For this review, use the dimensioned drawing (mm, ordinates from the lowest corner) and the shaded views. A direction names the side the tool comes from. Coordinates: 2 decimals unless noted, no trailing zeros. Order: outer loops, then holes, each group sorted by start corner. A loop starts at its lowest first (then second) coordinate and runs counter-clockwise, first axis right, second up. Notation, with made-up numbers: M 6,80 L 23,80 A20 cw 23,112 Z; hole C -39.75,47 d11. An arc over 180 degrees is marked long. Answer in a Markdown table with one row per item.
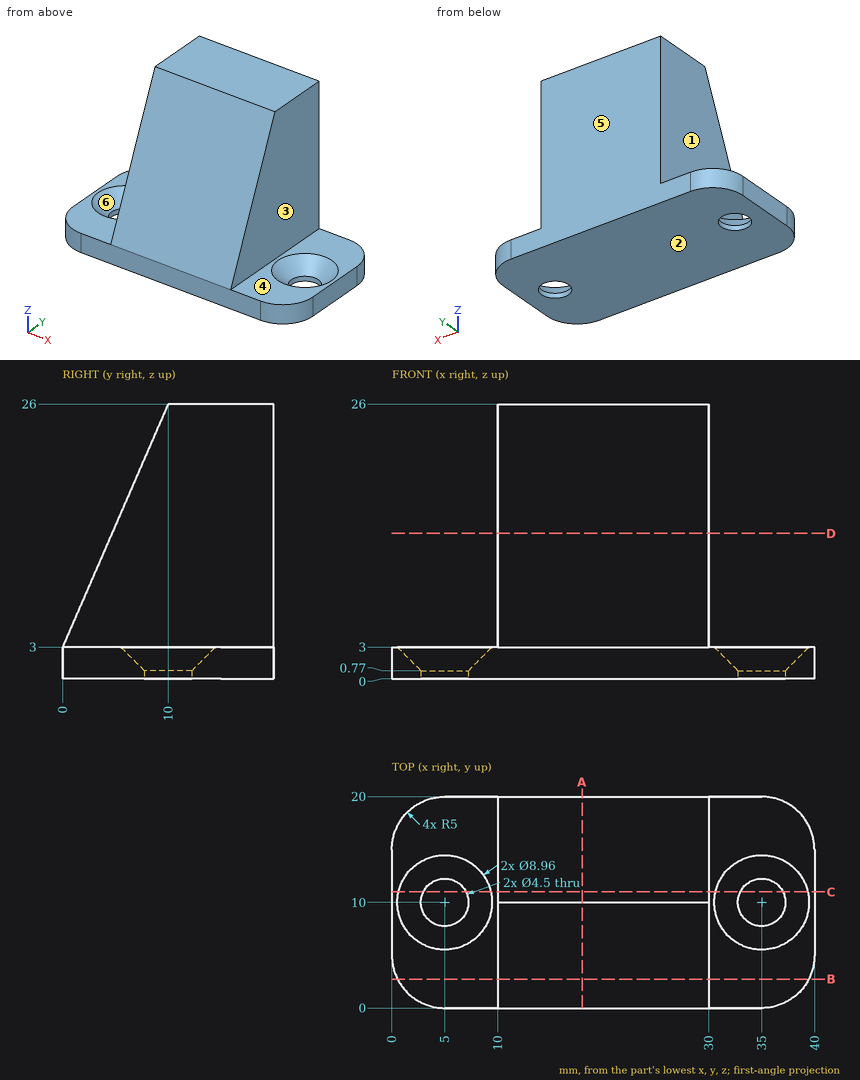
(1) Draft analysis for pull direction Y (two halves, no side actions). For the marked faces 4, 5 and 6, state which applies: pulls with the +Y half, pulls with the -Y half, needs draft (parallel to the pull), parting line crosses it, or undercut.
Return value:
| item | result |
|---|---|
| face 4 | needs draft |
| face 5 | pulls with the +Y half |
| face 6 | undercut |
(2) Add section A-A, the plane x = 18. Give the boundary of the cut face in (y, z), and give its area (3 significant figures).
Return value:
| item | result |
|---|---|
| outline | M 0,0 L 20,0 L 20,26 L 10,26 L 0,3 Z |
| area | 405 mm2 |
(3) For the marked faces 1, 2 and 3, list the 3-axis set-ups (+Z, -Z, +X, -X, +Y, -Y) from which the entire face can be reached by the end or side of a thin tool; tool diameter is ignored.
Return value:
| item | result |
|---|---|
| face 1 | +Z, -X, +Y, -Y |
| face 2 | -Z, +X, -X, +Y, -Y |
| face 3 | +Z, +X, +Y, -Y |
(4) Add section D-D, the plane z = 13.75. Give the boundary of the cut face in (x, y), and give its area (3 significant figures).
Return value:
| item | result |
|---|---|
| outline | M 10,4.67 L 30,4.67 L 30,20 L 10,20 Z |
| area | 307 mm2 |
(5) Insertion check: pin 1 Ø12 at (x, z) = (8, 11.5) entering from +Y; pin 2 Ø7 at (x, y) = (5, 10) entering from +Z; pin 3 Ø10 at (y, z) = (9.5, 18.5) entering from -X; pin 4 Ø6 at (x, y) = (35, 10) entering from +Z. Each pin has a flat end and moves straight along its axis. Give the tip position at first contact, or say it passes through.
Return value:
| item | result |
|---|---|
| pin 1 | stops at y = 20 |
| pin 2 | stops at z = 2.02 |
| pin 3 | stops at x = 10 |
| pin 4 | stops at z = 1.52 |
(6) Add section B-B, the plane y = 2.75. Give the boundary of the cut face in (x, z) (3 decimals), and give its area (3 significant figures).
Return value:
| item | result |
|---|---|
| outline | M 0.535,0 L 39.465,0 L 39.465,3 L 30,3 L 30,9.325 L 10,9.325 L 10,3 L 0.535,3 Z |
| area | 243 mm2 |
(7) Add section C-C, the plane y = 11. Give the number of separate pieces and of enclosed holes in the cut face, and give its area (3 significant figures).
Return value:
| item | result |
|---|---|
| separate pieces | 3 |
| enclosed holes | 0 |
| area | 545 mm2 |
(8) For line 1 along X through (y, z) = (10, 0.4); line 2 along Y through (x, z) = (35, 0.4); line 3 along Z through (x, y) = (35, 2.5), list the stretches that pass through material, from the lowest coordinate up. Write a range as from..to.
Return value:
| item | result |
|---|---|
| line 1 | x = 0..2.75, 7.25..32.75, 37.25..40 |
| line 2 | y = 0..7.75, 12.25..20 |
| line 3 | z = 0..3 |
